Could you check a few things on this model? Use its own coordinates, in mm. A direction names the side the tool comes from. Give positions to 0.01 mm unless a question says otherwise; leave off trailing zeros. Loops run counter-clockwise (first coordinate to the right, second up) from the corner with the lowest first, then second, coordinate; pieces in that order, holes last. Notation, with made-up numbers: (89.5, 18) - (108.5, 18) arc R18 ccw to (108.5, 25) - close; hole circle Ø8 at (-24.5, -12). An arc over 180 degrees is marked (long way). Write each question's results on one line, items separated by ' | '. Start each with the question number.
1) I want a section at A-A, the plane x = 0. Write out the boundary of the cut face in (y, z), and give its area (3 significant figures).
2) On a 3-axis mill with a long thin cutter (end or side, diameter ignored), from which of +Z, -Z, +X, -X, +Y, -Y can I reach the whole of each face in a straight line? I mean faces 1 (the face through (-16.5, 58, 2)), 2 (the face through (0, 56, 3.75)), 3 (the face through (16.5, 58, 2)). Say none if no direction works.
3) If I drill on probe 1 along X at (y, z) = (56, 3.1); probe 2 along Z at (x, y) = (-40, -24); probe 3 along Z at (x, y) = (-62, -19.5), over which ranges is the centre line in solid material (lowest first)? Write a range as [from, to].
4) I'm going to push a flat-ended pin straight in: pin 1 (1.1 mm diameter, centred on x = -1, z = 1, fed in from +Y). Where does the tip first touch, or does it pass through?
5) I want a section at B-B, the plane z = 0.85. Write out the boundary of the cut face in (x, y).
from build123d import *

# Parameters (mm, degrees)
F3_DEPTH = 22.5
F4_DEPTH = 3.75


with BuildPart() as f1:
    # F0 (on Front) → F1 (revolve)
    with BuildSketch(Plane.XZ):
        Polygon((0, 0), (0, 11.919704), (-67.6, 0), align=None)
    revolve(axis=Axis((0, 0, 5.959852), (0, 0, -1)))

    # F2 (on Top) → F3 (cut, symmetric)
    with BuildSketch(Plane.XY):
        with BuildLine():
            ThreePointArc((-16.5, 43.47413), (-26.410225, -38.272052), (46.5, 0))
            ThreePointArc((46.5, 0), (38.272052, 26.410225), (16.5, 43.47413))
            ThreePointArc((16.5, 43.47413), (0, 46.5), (-16.5, 43.47413))
        make_face()
    extrude(amount=F3_DEPTH, both=True, mode=Mode.SUBTRACT)

    # F2 (on Top) → F4 (join)
    with BuildSketch(Plane.XY):
        with BuildLine():
            ThreePointArc((-16.5, 43.47413), (0, 46.5), (16.5, 43.47413))
            Line((16.5, 43.47413), (16.5, 67.52056))
            Line((16.5, 67.52056), (-16.5, 67.52056))
            Line((-16.5, 67.52056), (-16.5, 43.47413))
        make_face()
    extrude(amount=F4_DEPTH)


solid = f1.part
Answers:
1) outline: (-67.6, 0) - (-46.5, 0) - (-46.5, 3.72) - close; (46.5, 0) - (67.6, 0) - (67.52, 0.01) - (67.52, 3.75) - (46.5, 3.75) - close | area: 118 mm2
2) face 1: +Z, -X, +Y | face 2: +Z, +X, -X, +Y, -Y | face 3: +Z, +X, +Y
3) probe 1: x = [-16.5, 16.5] | probe 2: z = [0, 3.69] | probe 3: z = [0, 0.46]
4) pin 1: stops at y = 67.52
5) outline: (-16.5, 60.57) arc R62.78 ccw (long way) to (16.5, 60.57) - (16.5, 67.52) - (-16.5, 67.52) - close; hole (-16.5, 43.47) arc R46.5 ccw (long way) to (46.5, 0) arc R46.5 ccw to (16.5, 43.47) arc R46.5 ccw to start
